Here's the drawing with two shaded views (mm, measured from the low corner). I have some questions. Round coordinates to 2 decimals unless told otherwise and drop trailing zeros. Loops run counter-clockwise (first coordinate to the right, second up) from the corner with the lowest first, then second, coordinate; pieces in that order, holes last. Notation, with made-up numbers: (-9, 84.25) -> (1, 84.25) arc R16 ccw to (1, 93.25) -> close; hole circle Ø8 at (-25.5, 24.25). An arc over 180 degrees is marked (long way). Write each question's results on one line, items separated by ' | '. Start each with the question number.
1) We'd pull the mould along Z, two halves only. Please class the marked faces 1, 2 and 3: pulls with the +Z half, pulls with the -Z half, needs draft (parallel to the pull), parting line crosses it, or undercut.
2) Imagine slicing it at D-D, the plane x = 1. List the corners of the cut face in (y, z) for me.
3) Imagine slicing it at C-C, the plane x = 8.5. List the corners of the cut face in (y, z) for me.
4) For P1, Ø1, axis at x = 4.5, y = 2, coming from the -Z side; P2, Ø1, axis at x = 2.5, z = 2.5, coming from the +Y side; P3, Ø2, axis at x = 3.5, z = 5.5, coming from the -Y side, each with a flat end and sliding along its axis, tell me the tip position at first contact or that it passes through.
5) If I drill on probe 1 along Y at (x, z) = (4.3, 4); probe 2 along X at (y, z) = (4, 2); probe 3 along Z at (x, y) = (3.5, 5.75) (1 decimal), over which ranges is the centre line in solid material (lowest first)?
6) Imagine slicing it at A-A, the plane z = 4. List the corners of the cut face in (x, y) for me.
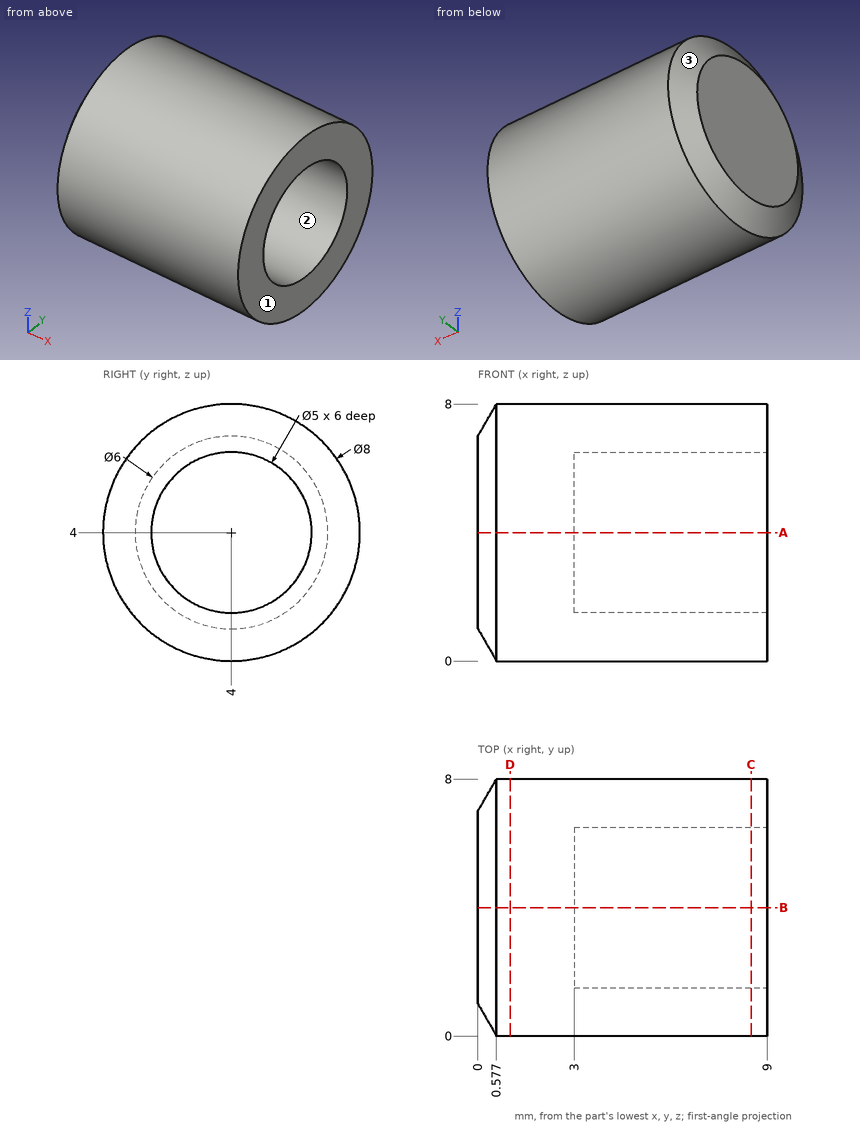
Checked values:
1) face 1: needs draft | face 2: undercut | face 3: parting line crosses it
2) outline: circle Ø8 at (4, 4)
3) outline: circle Ø8 at (4, 4); hole circle Ø5 at (4, 4)
4) P1: z = 0.29 | P2: y = 7.87 | P3: y = 0.03
5) probe 1: 0 to 1.5, 6.5 to 8 | probe 2: 0 to 3 | probe 3: 0.4 to 2.2, 5.8 to 7.6
6) outline: (0, 1) -> (0.58, 0) -> (9, 0) -> (9, 1.5) -> (3, 1.5) -> (3, 6.5) -> (9, 6.5) -> (9, 8) -> (0.58, 8) -> (0, 7) -> close
